from build123d import *

# Parameters (mm, degrees)
SKETCH_2_R                = 150
EXTRUDE_1_DEPTH           = 15
SKETCH_3_R                = 35
CUT_EXTRUDE_1_DEPTH       = 3
EXTRUDE_START             = 16.5
SKETCH_4_R                = 38.5
SKETCH_4_R_2              = 35
EXTRUDE_2_DEPTH           = 16.5
EXTRUDE_START_2           = 13.5
SKETCH_5_R                = 46.5
SKETCH_5_R_2              = 38.5
EXTRUDE_3_DEPTH           = 13.5
CHAMFER_1_SIZE            = 0.5
HOLE_WIZARD_1_D           = 6.6
HOLE_WIZARD_1_CBORE_D     = 11
HOLE_WIZARD_1_CBORE_DEPTH = 8
HOLE_WIZARD_6_0_6_1_D     = 6
CHAMFER_3_SIZE            = 1
CUT_EXTRUDE_START         = 69
SKETCH_20_R               = 46.5
CUT_EXTRUDE_5_DEPTH       = 69
SKETCH_22_R               = 4
CUT_EXTRUDE_7_DEPTH       = 244.812402925
CHAMFER_6_SIZE            = 1
HOLE_WIZARD_M8_1_D        = 6.8
EXTRUDE_START_3           = 5
SKETCH_27_R               = 40
SKETCH_27_R_2             = 35
EXTRUDE_4_DEPTH           = 5
CHAMFER_7_SIZE            = 0.5
CHAMFER_8_SIZE            = 2
SKETCH_25_R               = 20
CUT_EXTRUDE_8_DEPTH       = 245.171021663
CHAMFER_9_SIZE            = 2
FILLET_1_R                = 1


with BuildPart() as part:
    # 草图2 → 凸台-拉伸1 (new body)
    with BuildSketch(Plane.XY.offset(1)):
        with Locations((18.556612769, -25.522523089)):
            Circle(SKETCH_2_R)
    extrude(amount=EXTRUDE_1_DEPTH)

    # 草图3 → 切除-拉伸1 (cut)
    with BuildSketch(Plane(origin=(0, 0, 1), x_dir=(-1, 0, 0), z_dir=(0, 0, -1))):
        with Locations((-18.556612769, -25.522523089)):
            Circle(SKETCH_3_R)
    extrude(amount=-CUT_EXTRUDE_1_DEPTH, mode=Mode.SUBTRACT)

    # 草图4 → 凸台-拉伸2 (add)
    with BuildSketch(Plane(origin=(0, 0, 1), x_dir=(-1, 0, 0), z_dir=(0, 0, -1)).offset(EXTRUDE_START)):
        with Locations(Location((-18.556612769, -25.522523089, 0), (0, 0, 180))):
            Circle(SKETCH_4_R)
        with Locations((-18.556612769, -25.522523089)):
            Circle(SKETCH_4_R_2, mode=Mode.SUBTRACT)
    extrude(amount=-EXTRUDE_2_DEPTH)

    # 草图5 → 凸台-拉伸3 (add)
    with BuildSketch(Plane(origin=(0, 0, 1), x_dir=(-1, 0, 0), z_dir=(0, 0, -1)).offset(EXTRUDE_START_2)):
        with Locations(Location((-18.556612769, -25.522523089, 0), (0, 0, 180))):
            Circle(SKETCH_5_R)
        with Locations(Location((-18.556612769, -25.522523089, 0), (0, 0, 90))):
            Circle(SKETCH_5_R_2, mode=Mode.SUBTRACT)
    extrude(amount=-EXTRUDE_3_DEPTH)

    # 倒角1
    chamfer_1_edges = [part.edges().sort_by_distance(p)[0] for p in [
        (53.556612769, -25.522523089, -15.5),
        (-19.943387231, -25.522523089, -15.5),
    ]]
    chamfer(chamfer_1_edges, length=CHAMFER_1_SIZE)

    # 打孔尺寸根据内六角圆柱头螺钉的类型1 (through all)
    with Locations(Plane(origin=(42.626407432, -13.463363362, 16), x_dir=(1, 0, 0), z_dir=(0, 0, 1))):
        with Locations((-41.703352232, 12.211350104), (-6.436237094, 12.211350104), (4.461900826, -21.329669558), (-52.601490152, -21.329669558)):
            CounterBoreHole(HOLE_WIZARD_1_D / 2, HOLE_WIZARD_1_CBORE_D / 2, HOLE_WIZARD_1_CBORE_DEPTH)

    # Ø6.0 (6) 直径孔1 (through all)
    with Locations(Plane.XY.offset(16)):
        with Locations((18.556612769, -55.522523089)):
            Hole(HOLE_WIZARD_6_0_6_1_D / 2)

    # 倒角3
    chamfer_3_edges = [part.edges().sort_by_distance(p)[0] for p in [
        (21.556612769, -55.522523089, 16),
    ]]
    chamfer(chamfer_3_edges, length=CHAMFER_3_SIZE)

    # 草图20 → 切除-拉伸5 (cut)
    with BuildSketch(Plane(origin=(0, 0, 1), x_dir=(-1, 0, 0), z_dir=(0, 0, -1)).offset(CUT_EXTRUDE_START)):
        with Locations((-18.556612769, -25.522523089)):
            Circle(SKETCH_20_R)
    extrude(amount=-CUT_EXTRUDE_5_DEPTH, mode=Mode.SUBTRACT)

    # 草图22 → 切除-拉伸7 (cut, through all)
    with BuildSketch(Plane.XY.offset(16)):
        with Locations((-1.443387231, -68.522523089)):
            Circle(SKETCH_22_R)
        with Locations((38.556612769, -68.522523089)):
            Circle(SKETCH_22_R)
    extrude(amount=-CUT_EXTRUDE_7_DEPTH, mode=Mode.SUBTRACT)

    # 倒角6
    chamfer_6_edges = [part.edges().sort_by_distance(p)[0] for p in [
        (-5.443387231, -68.522523089, 16),
        (34.556612769, -68.522523089, 16),
    ]]
    chamfer(chamfer_6_edges, length=CHAMFER_6_SIZE)

    # M8 螺纹孔1 (through all)
    with Locations(Plane.XY.offset(16)):
        with Locations((-31.443387231, -43.522523089), (-31.443387231, -63.522523089), (68.556612769, -43.522523089), (68.556612769, -63.522523089), (18.556612769, -25.522523089)):
            Hole(HOLE_WIZARD_M8_1_D / 2)

    # 草图27 → 凸台-拉伸4 (add)
    with BuildSketch(Plane(origin=(0, 0, 1), x_dir=(-1, 0, 0), z_dir=(0, 0, -1)).offset(EXTRUDE_START_3)):
        with Locations(Location((-18.556612769, -25.522523089, 0), (0, 0, 180))):
            Circle(SKETCH_27_R)
        with Locations((-18.556612769, -25.522523089)):
            Circle(SKETCH_27_R_2, mode=Mode.SUBTRACT)
    extrude(amount=-EXTRUDE_4_DEPTH)

    # 倒角7
    chamfer_7_edges = [part.edges().sort_by_distance(p)[0] for p in [
        (53.556612769, -25.522523089, -4),
    ]]
    chamfer(chamfer_7_edges, length=CHAMFER_7_SIZE)

    # 倒角8
    chamfer_8_edges = [part.edges().sort_by_distance(p)[0] for p in [
        (-131.443387231, -25.522523089, 1),
        (-131.443387231, -25.522523089, 16),
    ]]
    chamfer(chamfer_8_edges, length=CHAMFER_8_SIZE)

    # 草图25 → 切除-拉伸8 (cut, through all)
    with BuildSketch(Plane.XY.offset(16)):
        with Locations((18.556612769, -25.522523089)):
            Circle(SKETCH_25_R)
    extrude(amount=-CUT_EXTRUDE_8_DEPTH, mode=Mode.SUBTRACT)

    # 倒角9
    chamfer_9_edges = [part.edges().sort_by_distance(p)[0] for p in [
        (-1.443387231, -25.522523089, 4),
        (-1.443387231, -25.522523089, 16),
    ]]
    chamfer(chamfer_9_edges, length=CHAMFER_9_SIZE)

    # 圆角1
    fillet_1_edges = [part.edges().sort_by_distance(p)[0] for p in [
        (-21.443387231, -25.522523089, 1),
    ]]
    fillet(fillet_1_edges, radius=FILLET_1_R)


solid = part.part
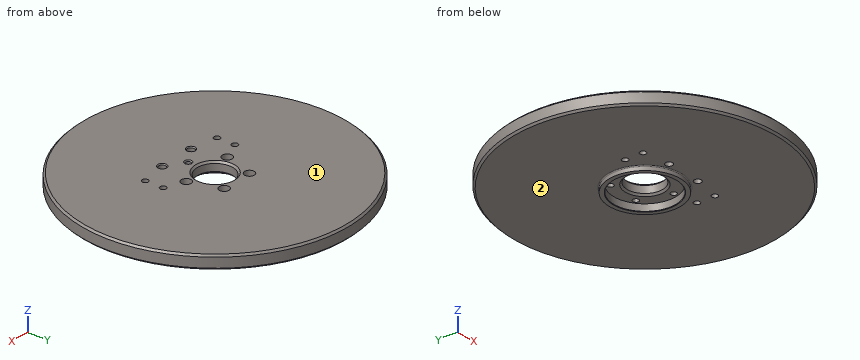
Model file for the job. Use its own axes, mm. Face numbers are marked on the shaded views. A direction names the side the tool comes from. Coordinates: 2 decimals unless noted, no trailing zeros. One line per item, written item: value. Start each with the question number.
1) Which spindle directions (+Z, -Z, +X, -X, +Y, -Y) get a long thin tool onto all of the face, cutting with end or side? Do the marked faces 1 and 2. Say none if no direction does.
2) Probe probe 1 along Y at (x, z) = (19, 8); probe 2 along Y at (x, z) = (-29.5, 9.5); probe 3 along Z at (x, y) = (64, -13.5). List the from-to ranges inside material, lowest first.
3) Flat gauge pins, fed straight in: pin 1 Ø9 at (x, y) = (0.5, 0) entering from +Z; pin 2 Ø10 at (y, z) = (27, 1.5) entering from +X; pin 3 Ø5.5 at (x, y) = (46.5, -37) entering from +Z; pin 4 Ø8.5 at (x, y) = (36.19, -1.25) entering from -Z. Where does each tip first touch, or does it go through?
Answers follow:
1. face 1: +Z, +X, -X, +Y, -Y
1. face 2: -Z
2. probe 1: -175.52 to -58.49, -52.56 to -45.52, -5.53 to 124.48
2. probe 2: -167.62 to -66.31, -60.73 to -46.31, -40.73 to 116.57
2. probe 3: 1 to 16
3. pin 1: z = 16
3. pin 2: x = 160.75
3. pin 3: z = 8
3. pin 4: z = 4
